from build123d import *

# Parameters (mm, degrees)
F0_W     = 40
F0_H     = 20
F1_DEPTH = 10
F2_R     = 2.75
F5_R     = 2.6
F7_R     = 4.65
F9_R     = 4.5


with BuildPart() as f1:
    # F0 (on Top) → F1 (new body)
    with BuildSketch(Plane.XY):
        Rectangle(F0_W, F0_H)
    extrude(amount=F1_DEPTH)

    # F2 (on face) → F6 section 0
    with BuildSketch(Plane.XY.offset(10)):
        with Locations((-10, 0)):
            Circle(F2_R)
    # F5 (on offset) → F6 section 1
    with BuildSketch(Plane.XY.offset(6.2)):
        with Locations((-10, 0)):
            Circle(F5_R)
    loft(mode=Mode.SUBTRACT)

    # F7 (on face) → F10 section 0
    with BuildSketch(Plane.XY.offset(10)):
        with Locations((10, 0)):
            Circle(F7_R)
    # F9 (on offset) → F10 section 1
    with BuildSketch(Plane.XY.offset(2.4)):
        with Locations((10, 0)):
            Circle(F9_R)
    loft(mode=Mode.SUBTRACT)


solid = f1.part
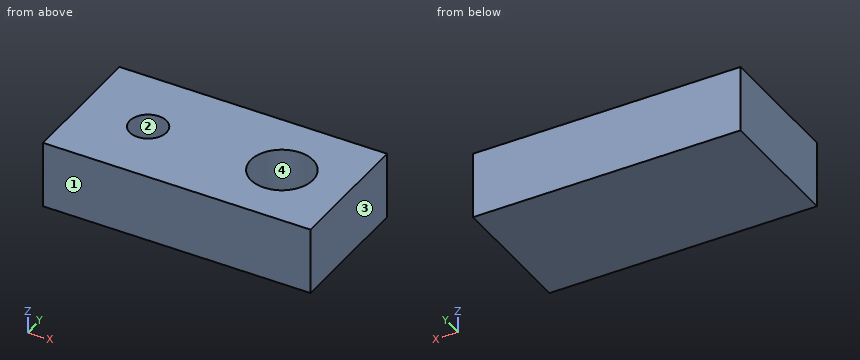
Part model, mm, in its own coordinate system. Face numbers are marked on the shaded views. Give positions to 0.01 mm unless a question says otherwise; leave off trailing zeros. Write each loop counter-clockwise with the first axis right and the second up, starting at its lowest first coordinate (ties: lowest second). Pieces come first, ordered by that corner, then holes.
1) Two-plate mould, pull along Y, no slides. Class the marked faces 1, 2, 3 and 4: released by +Y, released by -Y, zero draft, split by the parting line, or undercut.
Resolved:
face 1: released by -Y
face 2: undercut
face 3: zero draft
face 4: undercut
2) Cut at A-A on x = -10. Write the cut outline in (y, z).
Resolved:
outline: (-10, 0) - (10, 0) - (10, 10) - (2.75, 10) - (2.6, 6.2) - (-2.6, 6.2) - (-2.75, 10) - (-10, 10) - close
3) Cut at B-B on z = 4.75. Write the cut outline in (x, y), then the cut area to 3 significant figures.
Resolved:
outline: (-20, -10) - (20, -10) - (20, 10) - (-20, 10) - close; hole circle Ø9.09 at (10, 0)
area: 735 mm2
4) Probe L1, parallel to X at y = -1, z = 9; L2, parallel to X at y = -0.5, z = 3.5; L3, parallel to X at y = -3, z = 6.25. List the from-to ranges inside material, lowest first.
Resolved:
L1: x = -20 to -12.52, -7.48 to 5.48, 14.52 to 20
L2: x = -20 to 5.51, 14.49 to 20
L3: x = -20 to 6.54, 13.46 to 20
